Can you work these out from the model? Positions are in its coordinate system, mm. Face numbers are marked on the shaded views. Give positions to 0.01 mm unless a question says otherwise; leave off trailing zeros. Order: outer loops, then holes, each group sorted by start corner. A loop starts at its lowest first (then second) coordinate and runs counter-clockwise, first axis right, second up.
```python
from build123d import *

# Parameters (mm, degrees)
SKETCH1_W           = 1219.2
SKETCH1_H           = 609.6
BOSS_EXTRUDE1_DEPTH = 609.6
SKETCH2_R           = 152.4
BOSS_EXTRUDE2_DEPTH = 50.8
FILLET1_R           = 25.4


with BuildPart() as part:
    # Sketch1 → Boss-Extrude1 (new body)
    with BuildSketch(Plane(origin=(0, 0, 0), x_dir=(1, 0, 0), z_dir=(0, 1, 0))):
        Rectangle(SKETCH1_W, SKETCH1_H)
    extrude(amount=BOSS_EXTRUDE1_DEPTH)

    # Sketch2 → Boss-Extrude2 (add)
    with BuildSketch(Plane.XY.offset(304.8)):
        with Locations(Location((-304.8, 304.8, 0), (0, 0, 180))):
            Circle(SKETCH2_R)
        with Locations(Location((304.8, 304.8, 0), (0, 0, 180))):
            Circle(SKETCH2_R)
    extrude(amount=BOSS_EXTRUDE2_DEPTH)

    # Fillet1
    fillet1_edges = [part.edges().sort_by_distance(p)[0] for p in [
        (-152.4, 304.8, 355.6),
        (457.2, 304.8, 355.6),
    ]]
    fillet(fillet1_edges, radius=FILLET1_R)


solid = part.part
```
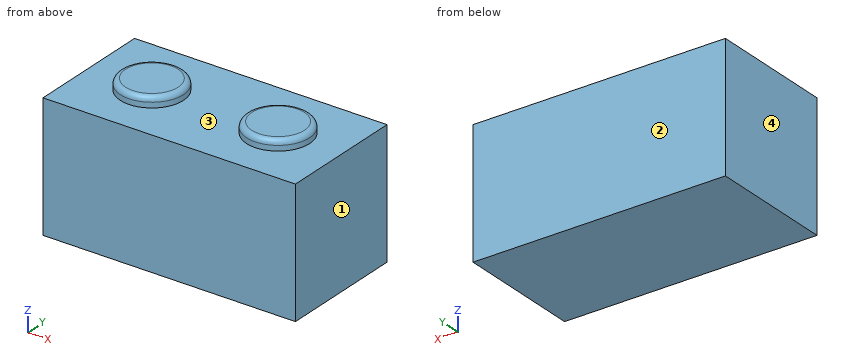
1) I'm going to push a flat-ended pin straight in: pin 1 Ø6 at (x, y) = (-446, 150) entering from +Z. Where does the tip first touch, or does it pass through?
2) Suppose I cut it at A-A (x = 304.8). Please give me the cut outline in (y, z), and give its area (3 significant figures).
3) Suppose I cut it at B-B (y = 304.8). Please give me the cut outline in (x, z).
4) We'd pull the mould along X, two halves only. Please class the marked faces 1, 2, 3 and 4: +X half, -X half, draft (parallel to the pull), parting line (faces both ways), or undercut.
5) Suppose I cut it at D-D (y = 127.5). Please give me the cut outline in (x, z), and give its area (3 significant figures).
6) If I drill on line 1 (Z direction, x = -453, y = 105), over which ranges is the centre line in solid material (lowest first)?
7) Suppose I cut it at C-C (x = -479.5). Please give me the cut outline in (y, z).
Results:
1. pin 1: stops at z = 304.8
2. outline: (0, -304.8) - (609.6, -304.8) - (609.6, 304.8) - (457.2, 304.8) - (457.2, 330.2) arc R25.4 ccw to (431.8, 355.6) - (177.8, 355.6) arc R25.4 ccw to (152.4, 330.2) - (152.4, 304.8) - (0, 304.8) - close
2. area: 387,000 mm2
3. outline: (-609.6, -304.8) - (609.6, -304.8) - (609.6, 304.8) - (457.2, 304.8) - (457.2, 330.2) arc R25.4 ccw to (431.8, 355.6) - (177.8, 355.6) arc R25.4 ccw to (152.4, 330.2) - (152.4, 304.8) - (-152.4, 304.8) - (-152.4, 330.2) arc R25.4 ccw to (-177.8, 355.6) - (-431.8, 355.6) arc R25.4 ccw to (-457.2, 330.2) - (-457.2, 304.8) - (-609.6, 304.8) - close
4. face 1: +X half
4. face 2: draft
4. face 3: undercut
4. face 4: -X half
5. outline: (-609.6, -304.8) - (609.6, -304.8) - (609.6, 304.8) - (-609.6, 304.8) - close
5. area: 743,000 mm2
6. line 1: z = -304.8 to 304.8
7. outline: (0, -304.8) - (609.6, -304.8) - (609.6, 304.8) - (0, 304.8) - close
